from build123d import *

# Parameters (mm, degrees)
F0_R          = 3.75
F1_DEPTH      = 2
F2_R          = 2.55
F3_DEPTH      = 25
F4_R          = 2.55
F5_DEPTH      = 25
F6_W          = 1.301092
F6_H          = 2.819048
F7_DEPTH      = 2
F8_W          = 2
F8_H          = 0.787675
F9_DEPTH      = 5
F9_DEPTH_BACK = 6


with BuildPart() as f1:
    # F0 (on Front) → F1 (new body)
    with BuildSketch(Plane.XZ):
        Circle(F0_R)
    extrude(amount=F1_DEPTH)

    # F2 (on Front) → F3 (cut)
    with BuildSketch(Plane.XZ):
        Circle(F2_R)
    extrude(amount=-F3_DEPTH, mode=Mode.SUBTRACT)

    # F4 (on face) → F5 (cut)
    with BuildSketch(Plane.XZ.offset(2)):
        Circle(F4_R)
    extrude(amount=-F5_DEPTH, mode=Mode.SUBTRACT)

    # F6 (on face) → F7 (join)
    with BuildSketch(Plane(origin=(0, 0, 0), x_dir=(-1, 0, 0), z_dir=(0, 1, 0))):
        with Locations((-0.162579, 4.866066)):
            Rectangle(F6_W, F6_H)
    extrude(amount=-F7_DEPTH)

    # F8 (on face) → F9 (join, two sides)
    with BuildSketch(Plane.YZ.offset(0.813125)) as f9_sk:
        with Locations((-1, 5.881752)):
            Rectangle(F8_W, F8_H)
    extrude(amount=F9_DEPTH)
    extrude(f9_sk.sketch, amount=-F9_DEPTH_BACK)


solid = f1.part
Geometry: final body of the model. Coordinates: model frame, mm. A direction names the side the tool comes from. Round coordinates to 2 decimals unless told otherwise and drop trailing zeros. Loops run counter-clockwise (first coordinate to the right, second up) from the corner with the lowest first, then second, coordinate; pieces in that order, holes last. Notation, with made-up numbers: (46, 6) - (101, 6) arc R21 ccw to (101, 36) - close; hole circle Ø4 at (14, 29.25). An arc over 180 degrees is marked (long way). Write each question's results on one line, items separated by ' | '. Start each with the question number.
1) Mould query, pull axis Z, two halves, no side actions, for faces 1 (the face through (-1, -2, 3)), 2 (the face through (-3, -1, 5.488)), 3 (the face through (-0.321, -0.986, -3.736)), 4 (the face through (-3, -1, 6.276)). Classes: released by +Z, released by -Z, zero draft, split by the parting line, or undercut.
2) First-contact query: P1, Ø4, axis at x = -1.5, z = -1.5, coming from the -Y side. Flat tip, straight axial feed; report the tip coordinate or a pass-through.
3) Cut plane C-C on y = -1. Return loops of the section in (x, z), then the cut area to 3 significant figures.
4) Cut plane A-A on x = 0. Return loops of the section in (y, z), then the cut area to 3 significant figures.
5) Cut plane D-D on x = 1.75. Return loops of the section in (y, z), then the cut area to 3 significant figures.
6) Cut plane B-B on z = 0. Return loops of the section in (x, y), then the cut area to 3 significant figures.
7) Access query for faces 5 (the face through (3, -1, 5.488)), 6 (the face through (-0.488, -1, 5)), 7 (the face through (3, -1, 6.276)). Directions: +Z, -Z, +X, -X, +Y, -Y. A direction counts if a zero-diameter tool reaches every point of the face in a straight line with its end or side. Return the directions, or none.
8) Line query: probe 1 along Z at (x, y) = (0, -1); probe 2 along Z at (x, y) = (1.75, -0.4); probe 3 along Z at (x, y) = (4.5, -0.7). Output: solid intervals per line, ascending. Write a range as [from, to].
Verdict:
1) face 1: zero draft | face 2: undercut | face 3: undercut | face 4: released by +Z
2) P1: stops at y = -2
3) outline: (-5.19, 5.49) - (-0.49, 5.49) - (-0.49, 3.72) arc R3.75 ccw (long way) to (0.81, 3.66) - (0.81, 5.49) - (5.81, 5.49) - (5.81, 6.28) - (-5.19, 6.28) - close; hole circle Ø5.1 at (0, 0) | area: 34.7 mm2
4) outline: (-2, -3.75) - (0, -3.75) - (0, -2.55) - (-2, -2.55) - close; (-2, 2.55) - (0, 2.55) - (0, 6.28) - (-2, 6.28) - close | area: 9.85 mm2
5) outline: (-2, -3.32) - (0, -3.32) - (0, -1.85) - (-2, -1.85) - close; (-2, 1.85) - (0, 1.85) - (0, 3.32) - (-2, 3.32) - close; (-2, 5.49) - (0, 5.49) - (0, 6.28) - (-2, 6.28) - close | area: 7.42 mm2
6) outline: (-3.75, -2) - (-2.55, -2) - (-2.55, 0) - (-3.75, 0) - close; (2.55, -2) - (3.75, -2) - (3.75, 0) - (2.55, 0) - close | area: 4.80 mm2
7) face 5: +X, +Y, -Y | face 6: -X, +Y, -Y | face 7: +Z, +X, -X, +Y, -Y
8) probe 1: z = [-3.75, -2.55], [2.55, 6.28] | probe 2: z = [-3.32, -1.85], [1.85, 3.32], [5.49, 6.28] | probe 3: z = [5.49, 6.28]
